Part model, mm, in its own coordinate system. Give positions to 0.01 mm unless a question says otherwise; leave off trailing zeros. Write each loop counter-clockwise with the first axis right and the second up, starting at its lowest first coordinate (ties: lowest second). Pieces come first, ordered by that corner, then holes. Notation, with made-up numbers: M 35,-35 L 59,-35 A5 cw 59,-30 Z; hole C 57,-24 d6. An arc over 180 degrees is marked long. Use a Markdown table: item, result.
Autodesk Inventor part; units mm, degrees
ref_plane "YZ Plane" through (0, 0, 0) normal (1, 0, 0) x (0, 1, 0)
ref_plane "XZ Plane" through (0, 0, 0) normal (0, 1, 0) x (-1, 0, 0)
ref_plane "XY Plane" through (0, 0, 0) normal (0, 0, 1) x (1, 0, 0)
sketch "Sketch1" plane through (0, 0, 0) normal (1, 0, 0) x (0, 1, 0)
  line L0 (46.0375, 63.5) -> (-46.0375, 63.5)
  line L1 (-46.0375, 63.5) -> (-46.0375, -63.5)
  line L2 (-46.0375, -63.5) -> (46.0375, -63.5)
  line L3 (46.0375, -63.5) -> (46.0375, 63.5)
  line L4 (46.0375, 63.5) -> (-46.0375, -63.5) construction
  line L5 (-46.0375, 63.5) -> (46.0375, -63.5) construction
  circle A0 centre (0, 0) radius 38.1
  dimension "d0" = 92.075
  dimension "d1" = 127
  dimension "d4" = 76.2
extrude "Extrusion1" add sketch "Sketch1" along normal blind 19.05
1. Cut at C-C, the plane x = 4.25. Give the cut face in (y, z).
Findings below:
| item | result |
|---|---|
| outline | M -46.04,-63.5 L 46.04,-63.5 L 46.04,63.5 L -46.04,63.5 Z; hole C 0,0 d76.2 |
2. Cut at A-A, the plane z = 0. Give the cut face in (x, y).
Findings below:
| item | result |
|---|---|
| outline | M 0,-46.04 L 19.05,-46.04 L 19.05,-38.1 L 0,-38.1 Z; M 0,38.1 L 19.05,38.1 L 19.05,46.04 L 0,46.04 Z |
3. Drill centre lines: L1, parallel to Z at x = 6.5, y = 0; L2, parallel to Y at x = 13.75, z = -2.5; L3, parallel to Z at x = 10.5, y = 31. Where is each one in solid material? Low to high.
Findings below:
| item | result |
|---|---|
| L1 | -63.5 to -38.1, 38.1 to 63.5 |
| L2 | -46.04 to -38.02, 38.02 to 46.04 |
| L3 | -63.5 to -22.15, 22.15 to 63.5 |
4. Cut at B-B, the plane y = 0. Give the cut face in (x, z), then the cut area to 3 significant figures.
Findings below:
| item | result |
|---|---|
| outline | M 0,-63.5 L 19.05,-63.5 L 19.05,-38.1 L 0,-38.1 Z; M 0,38.1 L 19.05,38.1 L 19.05,63.5 L 0,63.5 Z |
| area | 968 mm2 |
5. Two-plate mould, pull along Z, no slides. Class faces 1 (the flat face through (9, 46.038, -1)), 2 (the cylindrical face through (9.392, -30.235, 23.183)), 3 (the flat face through (9, -1, -63.5)), 4 (the flat face through (9, 1, 63.5)): released by +Z, released by -Z, zero draft, split by the parting line, or undercut.
Findings below:
| item | result |
|---|---|
| face 1 | zero draft |
| face 2 | undercut |
| face 3 | released by -Z |
| face 4 | released by +Z |
